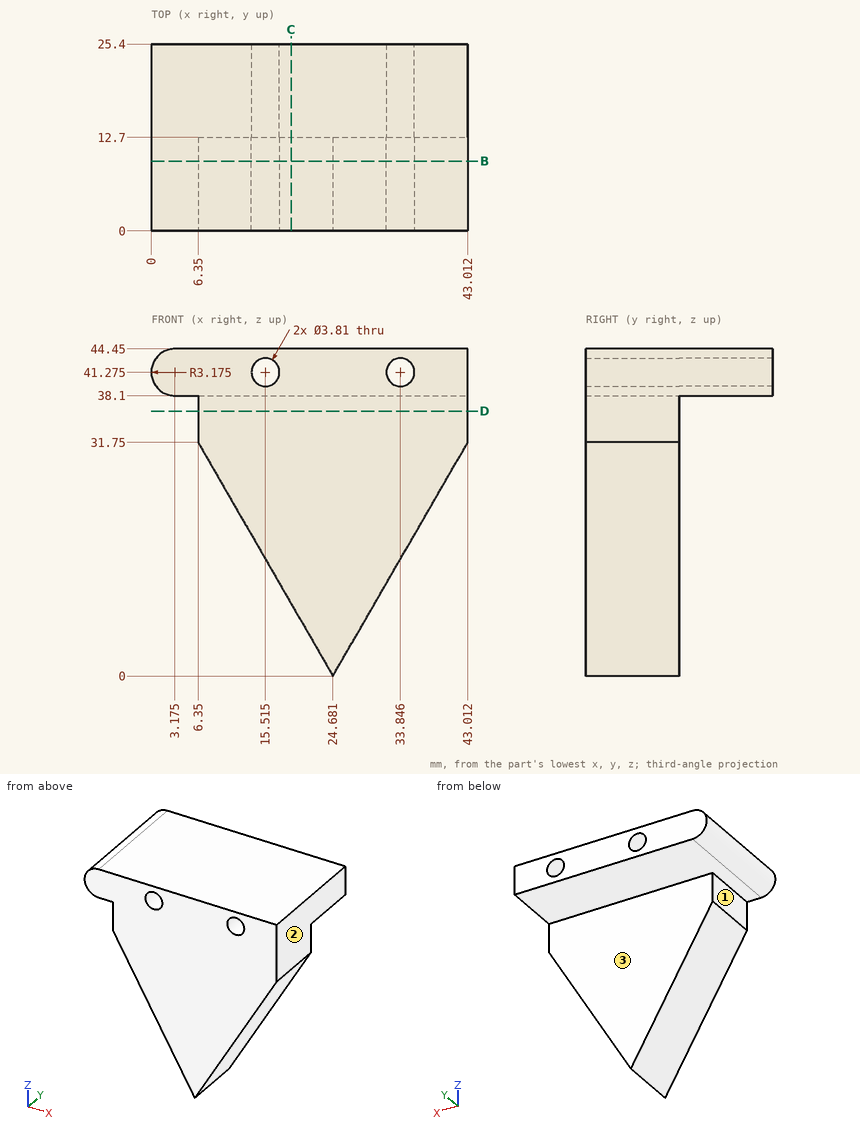
Input: dimensioned drawing with shaded views. Units: mm. Origin: part minimum x, y, z. A direction names the side the tool comes from. Give positions to 0.01 mm unless a question says otherwise; leave off trailing zeros. Write each loop counter-clockwise with the first axis right and the second up, starting at its lowest first coordinate (ties: lowest second). Pieces come first, ordered by that corner, then holes.
Q1. Set-up query: the marked faces 1, 2 and 3. Return all of +Z, -Z, +X, -X, +Y, -Y with unobstructed straight access to the full face (end or side cutting, diameter ignored); none if empty.
Q2. Section C-C, the plane x = 19. Output: boundary loops of the cut face in (y, z), plus the area to 3 significant figures.
Q3. Section D-D, the plane z = 36. Output: boundary loops of the cut face in (x, y), plus the area to 3 significant figures.
Q4. First-contact query: P1, Ø12, axis at x = 29, y = 22.5, coming from the -Z side; P2, Ø2, axis at y = 10, z = 21.5, coming from the -X side; P3, Ø11, axis at x = 29.5, z = 11, coming from the +Y side. Flat tips, straight axial feed; report the tip coordinate or a pass-through.
Q5. Section B-B, the plane y = 9.5. State how many separate pieces and enclosed holes the cut face has, plus the area to 3 significant figures.
Q6. Material intervals for probe 1 along X at (y, z) = (21.75, 40.5) (1 decimal); probe 2 along Y at (x, z) = (16, 23); probe 3 along Z at (x, y) = (13.5, 15.25), sorted ascending.
Filled in:
1. face 1: -Z, -X, +Y, -Y
1. face 2: +Z, -Z, +X, +Y, -Y
1. face 3: -Z, +X, -X, +Y
2. outline: (0, 9.84) - (12.7, 9.84) - (12.7, 38.1) - (25.4, 38.1) - (25.4, 44.45) - (0, 44.45) - close
2. area: 520 mm2
3. outline: (6.35, 0) - (43.01, 0) - (43.01, 12.7) - (6.35, 12.7) - close
3. area: 466 mm2
4. P1: stops at z = 38.1
4. P2: stops at x = 11.69
4. P3: stops at y = 12.7
5. separate pieces: 1
5. enclosed holes: 2
5. area: 1,060 mm2
6. probe 1: x = 0.1 to 13.8, 17.3 to 32.1, 35.6 to 43
6. probe 2: y = 0 to 12.7
6. probe 3: z = 38.1 to 44.45
